```python
from build123d import *


with BuildPart() as part:
    # Sketch1 → Revolve1 (revolve)
    with BuildSketch(Plane.XY):
        with BuildLine():
            Line((-70.664700289, -47.5), (-65.664700289, -47.5))
            Line((-65.664700289, -47.5), (-65.664700289, -40))
            Line((-65.664700289, -40), (-53.033215522, -40))
            Line((-53.033215522, -40), (-53.033215522, -37))
            Line((-53.033215522, -37), (-49.033215522, -37))
            Line((-49.033215522, -37), (-49.033215522, -40))
            Line((-49.033215522, -40), (-43.588058898, -40))
            ThreePointArc((-43.588058898, -40), (-43.234505508, -39.853553391), (-43.088058898, -39.5))
            Line((-43.088058898, -39.5), (-43.088058898, -34.5))
            ThreePointArc((-43.088058898, -34.5), (-42.941612289, -34.146446609), (-42.588058898, -34))
            Line((-42.588058898, -34), (-37.50828788, -34))
            Line((-37.50828788, -34), (-37.50828788, -30))
            Line((-37.50828788, -30), (-39.064374409, -30))
            Line((-39.064374409, -30), (-39.064374409, -31.5))
            Line((-39.064374409, -31.5), (-44.064374409, -31.5))
            Line((-44.064374409, -31.5), (-44.064374409, -30))
            Line((-44.064374409, -30), (-57.429010066, -30))
            Line((-57.429010066, -30), (-57.429010066, -33))
            Line((-57.429010066, -33), (-62.429010066, -33))
            Line((-62.429010066, -33), (-62.429010066, -30))
            Line((-62.429010066, -30), (-66.725082253, -30))
            Line((-66.725082253, -30), (-66.725082253, -33))
            Line((-66.725082253, -33), (-69.725082253, -33))
            Line((-69.725082253, -33), (-69.725082253, -30))
            Line((-69.725082253, -30), (-70.664700289, -30))
            Line((-70.664700289, -30), (-70.664700289, -47.5))
        make_face()
    revolve(axis=Axis((-81.578167515, 0, 0), (1, 0, 0)))


solid = part.part
```
CAD build for the part. Positions are in the model's coordinates, mm. A direction names the side the tool comes from. Coordinates: 2 decimals unless noted, no trailing zeros. Loops run counter-clockwise (first coordinate to the right, second up) from the corner with the lowest first, then second, coordinate; pieces in that order, holes last. Notation, with made-up numbers: (-34.5, 23) - (7.5, 23) arc R35 cw to (7.5, 55) - close; hole circle Ø5 at (72.5, 50). An arc over 180 degrees is marked (long way). Return JSON: item names as keys, results as strings.
1. 3-axis set-ups, long thin cutter, end or side, ignore diameter. For faces 1 (the flat face through (-53.033, -11.7, 35.4)), 2 (the cylindrical face through (-64.61, 29.97, -1.32)), 3 (the cylindrical face through (-59.26, 8.67, 39.05)): which of +Z, -Z, +X, -X, +Y, -Y reach the whole face in a straight line?
Result:
{"face 1": "none", "face 2": "+X, -X", "face 3": "+X"}
2. Band-saw the part on A-A (x = -55.5). Give the cut face in (y, z), and give its area (3 significant figures).
Result:
{"outline": "circle Ø80 at (0, 0); hole circle Ø60 at (0, 0)", "area": "2,200 mm2"}
3. Drop flat-ended pins along their axis: pin 1 (6 mm diameter, centred on x = -50.5, y = 21, fed in from +Z); pin 2 (8 mm diameter, centred on x = -46, y = 14, fed in from +Z); pin 3 (10 mm diameter, centred on x = -44.5, z = -1.5, fed in from +Y); pin 4 (2 mm diameter, centred on y = 25, z = -12.5, fed in from -X). Give the stop position or say it passes through.
Result:
{"pin 1": "stops at z = 35.53", "pin 2": "stops at z = 38.73", "pin 3": "stops at y = 40", "pin 4": "passes through"}
4. Band-saw the part on B-B (z = 41.5). Give the cut face in (x, y), and give its area (3 significant figures).
Result:
{"outline": "(-70.66, -23.11) - (-65.66, -23.11) - (-65.66, 23.11) - (-70.66, 23.11) - close", "area": "231 mm2"}
5. Probe L1, parallel to Z at x = -60.4, y = 0; L2, parallel to Z at x = -41.8, y = 0. List the from-to ranges inside material, lowest first. Write a range as from..to.
Result:
{"L1": "z = -40..-33, 33..40", "L2": "z = -34..-31.5, 31.5..34"}
6. Band-saw the part on C-C (x = -41). Give the cut face in (y, z), and give its area (3 significant figures).
Result:
{"outline": "circle Ø68 at (0, 0); hole circle Ø63 at (0, 0)", "area": "514 mm2"}
7. Mould opens along X. For faces 4 (the flat face through (-49.033, 11.7, 35.4)), 5 (the cylindrical face through (-70.2, 29.97, -1.32)), 6 (the cylindrical face through (-41.599, 4.101, -31.232)), 7 (the flat face through (-37.508, -2.4, 30.1)) say: released by +X, released by -X, zero draft, split by the parting line, or undercut.
Result:
{"face 4": "undercut", "face 5": "zero draft", "face 6": "undercut", "face 7": "released by +X"}
